```python
from build123d import *

# Parameters (mm, degrees)
CROQUIS1_R              = 1.5000002
CROQUIS1_R_2            = 1.49999991
SALIENTE_EXTRUIR1_DEPTH = 8


with BuildPart() as part:
    # Croquis1 → Saliente-Extruir1 (new body)
    with BuildSketch(Plane(origin=(0, 0, 0), x_dir=(1, 0, 0), z_dir=(0, 1, 0))):
        with BuildLine():
            Line((-1.19757039, -21.678985349), (7.496084148, -0.648595564))
            Line((7.496084148, -0.648595564), (7.496084148, 24.351404436))
            Line((7.496084148, 24.351404436), (0.996084148, 24.351404436))
            Line((0.996084148, 24.351404436), (0.996084148, -0.648595564))
            Line((0.996084148, -0.648595564), (-0.503915852, -0.648595564))
            Line((-0.503915852, -0.648595564), (-6.872429124, -19.740170948))
            ThreePointArc((-6.872429124, -19.740170948), (-4.970266204, -23.44707843), (-1.19757039, -21.678985349))
        make_face()
        with Locations((1.996084371, -3.648597796)):
            Circle(CROQUIS1_R, mode=Mode.SUBTRACT)
        with Locations((-4.003916027, -20.618596904)):
            Circle(CROQUIS1_R_2, mode=Mode.SUBTRACT)
    extrude(amount=SALIENTE_EXTRUIR1_DEPTH)


solid = part.part
```
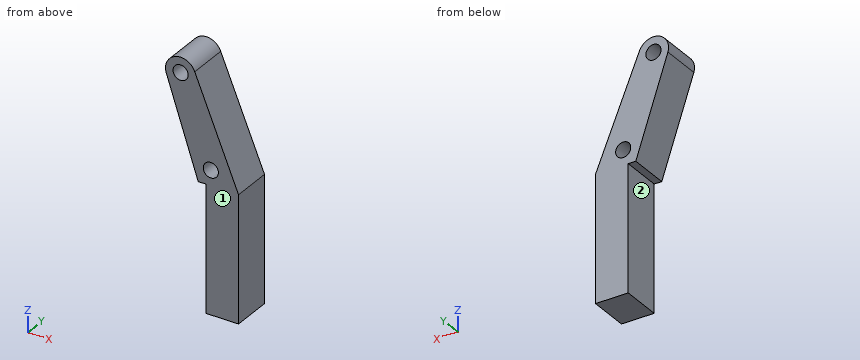
Source: CAD feature listing. Evaluate the final solid. Frame: model axes, mm. Face numbers are marked on the shaded views. A direction names the side the tool comes from. Round coordinates to 2 decimals unless told otherwise and drop trailing zeros. Loops run counter-clockwise (first coordinate to the right, second up) from the corner with the lowest first, then second, coordinate; pieces in that order, holes last. Notation, with made-up numbers: M 81.5,22.5 L 127.5,22.5 A29 ccw 127.5,46.5 Z; hole C -32.5,79 d9. An arc over 180 degrees is marked long. Put each result on its own line as item: value.
(1) First-contact query: pin 1 (1.2 mm diameter, centred on x = 0, y = 6, fed in from -Z); pin 2 (3 mm diameter, centred on y = 2, z = -11.5, fed in from -X); pin 3 (1.5 mm diameter, centred on x = -0.5, y = 5.5, fed in from +Z). Flat tips, straight axial feed; report the tip coordinate or a pass-through.
Solutions:
pin 1: z = 0.65
pin 2: x = 1
pin 3: z = 21.81
(2) Section B-B, the plane z = 4.5. Return loops of the section in (x, y), and give its area (3 significant figures).
Solutions:
outline: M -1.79,0 L 0.76,0 L 0.76,8 L -1.79,8 Z; M 3.23,0 L 5.9,0 L 5.9,8 L 3.23,8 Z
area: 41.8 mm²
(3) Section A-A, the plane x = 2.5. Return loops of the section in (y, z), and give its area (3 significant figures).
Solutions:
outline: M 0,-24.35 L 8,-24.35 L 8,2.24 L 0,2.24 Z; M 0,5.06 L 8,5.06 L 8,12.73 L 0,12.73 Z
area: 274 mm²
(4) Section C-C, the plane y = 5.75. Return loops of the section in (x, z), and give its area (3 significant figures).
Solutions:
outline: M -6.87,19.74 L -0.5,0.65 L 1,0.65 L 1,-24.35 L 7.5,-24.35 L 7.5,0.65 L -1.2,21.68 A3 ccw Z; hole C -4,20.62 d3; hole C 2,3.65 d3
area: 306 mm²
(5) Section D-D, the plane x = 5. Return loops of the section in (y, z), and give its area (3 significant figures).
Solutions:
outline: M 0,-24.35 L 8,-24.35 L 8,6.69 L 0,6.69 Z
area: 248 mm²
(6) Access query for the marked faces 1 and 2. Directions: +Z, -Z, +X, -X, +Y, -Y. A direction counts if a zero-diameter tool reaches every point of the face in a straight line with its end or side. Return the directions, or none.
Solutions:
face 1: +Z, -Z, +X, -X, -Y
face 2: -Z, -X, +Y, -Y
(7) Ray query, line 1 (Z direction, x = 1.75, y = 3); line 2 (X direction, y = 5.75, z = -8.5); line 3 (Z direction, x = 2.5, y = 0.75). Return the intervals inside material, ascending. Write a range as [from, to].
Solutions:
line 1: [-24.35, 2.17], [5.13, 14.55]
line 2: [1, 7.5]
line 3: [-24.35, 2.24], [5.06, 12.73]
